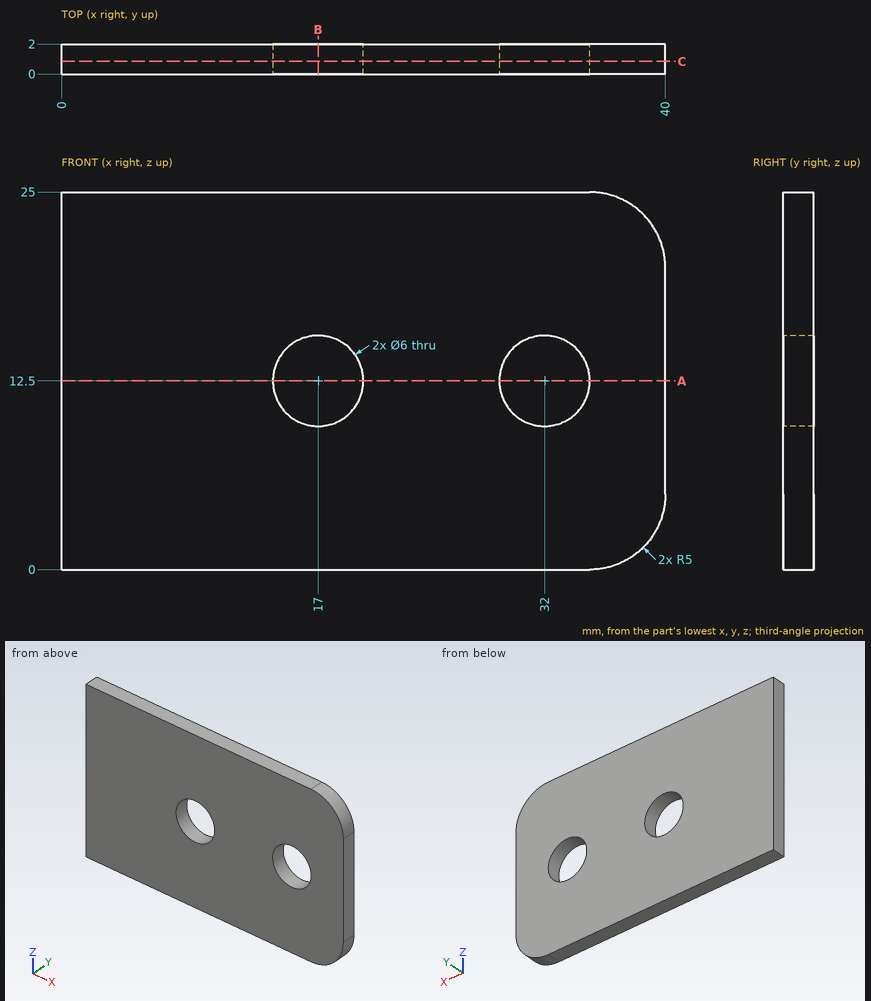
Could you check a few things on this drawing? It's one solid part, dimensions in mm from its lowest x, y, z. Round coordinates to 2 decimals unless told otherwise and drop trailing zeros. Order: outer loops, then holes, each group sorted by start corner. A loop starts at its lowest first (then second) coordinate and runs counter-clockwise, first axis right, second up. Notation, with made-up numbers: M 71,36 L 85,36 A30 ccw 85,65 Z; hole C -6,-27.5 d9. An arc over 180 degrees is marked long. Return JSON: item names as keys, results as strings. Group by question number.
1. If we section it at C-C on y = 0.85: List the corners of the cut face in (x, z) for me.
2. If we section it at A-A on z = 12.5: List the corners of the cut face in (x, y) for me, then the cut area to 3 significant figures.
3. Please list where these lines run through material, in increasing order: probe 1 along Z at (x, y) = (32, 1); probe 2 along X at (y, z) = (0.85, 13); probe 3 along X at (y, z) = (0.45, 9.75).
4. If we section it at B-B on x = 17: List the corners of the cut face in (y, z) for me.
Reply:
{
 "1": {"outline": "M 0,0 L 35,0 A5 ccw 40,5 L 40,20 A5 ccw 35,25 L 0,25 Z; hole C 17,12.5 d6; hole C 32,12.5 d6"},
 "2": {"outline": "M 0,0 L 14,0 L 14,2 L 0,2 Z; M 20,0 L 29,0 L 29,2 L 20,2 Z; M 35,0 L 40,0 L 40,2 L 35,2 Z", "area": "56.0 mm^2"},
 "3": {"probe 1": "0 to 9.5, 15.5 to 25", "probe 2": "0 to 14.04, 19.96 to 29.04, 34.96 to 40", "probe 3": "0 to 15.8, 18.2 to 30.8, 33.2 to 40"},
 "4": {"outline": "M 0,0 L 2,0 L 2,9.5 L 0,9.5 Z; M 0,15.5 L 2,15.5 L 2,25 L 0,25 Z"}
}
